from build123d import *

# Parameters (mm, degrees)
CROQUIS1_R              = 44.9
SALIENTE_EXTRUIR1_DEPTH = 3


with BuildPart() as part:
    # Croquis1 → Saliente-Extruir1 (new body)
    with BuildSketch(Plane.XY):
        Circle(CROQUIS1_R)
        with BuildLine():
            Line((-2.5, 33.907963666), (-2.5, 34.81034329))
            ThreePointArc((-2.5, 34.81034329), (-13.35565179, 32.243395685), (-22.846862843, 26.382396749))
            Line((-22.846862843, 26.382396749), (-22.208784092, 25.744317998))
            ThreePointArc((-22.208784092, 25.744317998), (-24.04163056, 24.04163056), (-25.744317998, 22.208784092))
            Line((-25.744317998, 22.208784092), (-26.382396749, 22.846862843))
            ThreePointArc((-26.382396749, 22.846862843), (-32.243395685, 13.35565179), (-34.81034329, 2.5))
            Line((-34.81034329, 2.5), (-33.907963666, 2.5))
            ThreePointArc((-33.907963666, 2.5), (-34, 0), (-33.907963666, -2.5))
            Line((-33.907963666, -2.5), (-34.81034329, -2.5))
            ThreePointArc((-34.81034329, -2.5), (-32.243395685, -13.35565179), (-26.382396749, -22.846862843))
            Line((-26.382396749, -22.846862843), (-25.744317998, -22.208784092))
            ThreePointArc((-25.744317998, -22.208784092), (-24.04163056, -24.04163056), (-22.208784092, -25.744317998))
            Line((-22.208784092, -25.744317998), (-22.846862843, -26.382396749))
            ThreePointArc((-22.846862843, -26.382396749), (-13.35565179, -32.243395685), (-2.5, -34.81034329))
            Line((-2.5, -34.81034329), (-2.5, -33.907963666))
            ThreePointArc((-2.5, -33.907963666), (0, -34), (2.5, -33.907963666))
            Line((2.5, -33.907963666), (2.5, -34.81034329))
            ThreePointArc((2.5, -34.81034329), (13.35565179, -32.243395685), (22.846862843, -26.382396749))
            Line((22.846862843, -26.382396749), (22.208784092, -25.744317998))
            ThreePointArc((22.208784092, -25.744317998), (24.04163056, -24.04163056), (25.744317998, -22.208784092))
            Line((25.744317998, -22.208784092), (26.382396749, -22.846862843))
            ThreePointArc((26.382396749, -22.846862843), (32.243395685, -13.35565179), (34.81034329, -2.5))
            Line((34.81034329, -2.5), (33.907963666, -2.5))
            ThreePointArc((33.907963666, -2.5), (34, 0), (33.907963666, 2.5))
            Line((33.907963666, 2.5), (34.81034329, 2.5))
            ThreePointArc((34.81034329, 2.5), (32.243395685, 13.35565179), (26.382396749, 22.846862843))
            Line((26.382396749, 22.846862843), (25.744317998, 22.208784092))
            ThreePointArc((25.744317998, 22.208784092), (24.04163056, 24.04163056), (22.208784092, 25.744317998))
            Line((22.208784092, 25.744317998), (22.846862843, 26.382396749))
            ThreePointArc((22.846862843, 26.382396749), (13.35565179, 32.243395685), (2.5, 34.81034329))
            Line((2.5, 34.81034329), (2.5, 33.907963666))
            ThreePointArc((2.5, 33.907963666), (0, 34), (-2.5, 33.907963666))
        make_face(mode=Mode.SUBTRACT)
    extrude(amount=SALIENTE_EXTRUIR1_DEPTH)


solid = part.part
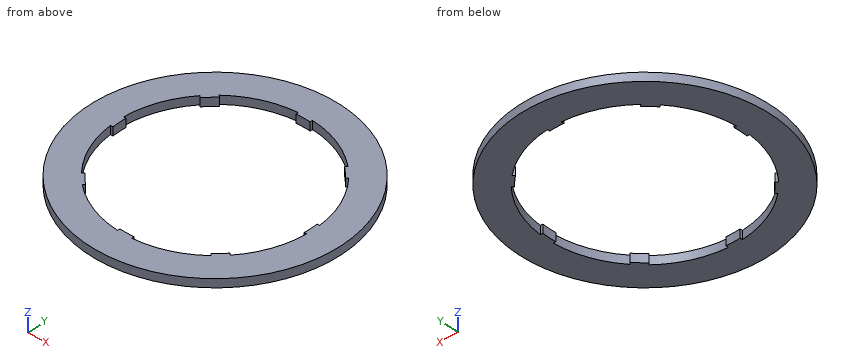
CAD build for the part. Positions are in the model's coordinates, mm. Coordinates: 2 decimals unless noted, no trailing zeros. Loops run counter-clockwise (first coordinate to the right, second up) from the corner with the lowest first, then second, coordinate; pieces in that order, holes last. Notation, with made-up numbers: (3.5, 72) - (14.5, 72) arc R18 ccw to (14.5, 80) - close; hole circle Ø6 at (-28, 77.5). An arc over 180 degrees is marked (long way). Use one line per item in the form item = value. Start each with the question number.
1) Drill centre lines: L1, parallel to X at y = 0.5, z = 1.45; L2, parallel to X at y = -22, z = 1.35; L3, parallel to Y at x = 24.5, z = 0.75. Where is each one in solid material? Low to high. Write a range as from..to.
2) Band-saw the part on A-A (y = 0). Give the cut face in (x, z).
3) Flat gauge pins, fed straight in: pin 1 (6 mm diameter, centred on x = -30, y = -6, fed in from -Z); pin 2 (0.7 mm diameter, centred on y = -34.5, z = 1, fed in from +X); pin 3 (1.5 mm diameter, centred on x = 29, z = 0.5, fed in from +Y); pin 4 (0.5 mm diameter, centred on x = -34.5, z = 2, fed in from -Y). Where does each tip first touch, or does it go through?
Check values:
q1.L1 = -44.9..-34, 34..44.9
q1.L2 = -39.14..-27.09, 27.09..39.14
q1.L3 = -37.63..-23.57, 23.57..37.63
q2.outline = (-44.9, 0) - (-34, 0) - (-34, 3) - (-44.9, 3) - close; (34, 0) - (44.9, 0) - (44.9, 3) - (34, 3) - close
q3.pin_1 = through
q3.pin_2 = 29.15
q3.pin_3 = 34.9
q3.pin_4 = -29.03
